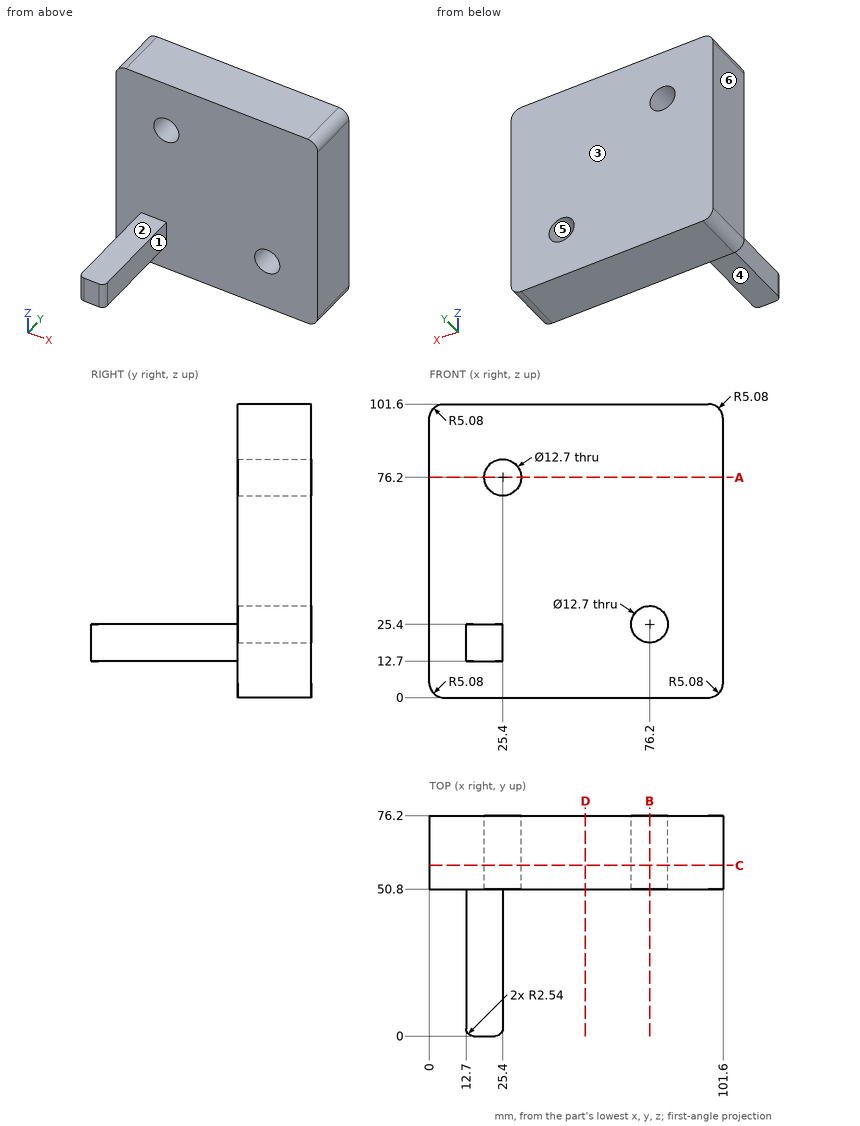
For this review, use the dimensioned drawing (mm, ordinates from the lowest corner) and the shaded views. A direction names the side the tool comes from. Round coordinates to 2 decimals unless told otherwise and drop trailing zeros. Loops run counter-clockwise (first coordinate to the right, second up) from the corner with the lowest first, then second, coordinate; pieces in that order, holes last. Notation, with made-up numbers: (-30.5, 77) -> (-7.5, 77) arc R15 ccw to (-7.5, 102) -> close; hole circle Ø3 at (-37.5, -32). An arc over 180 degrees is marked (long way). Write item = value, one per line. Start each with the question number.
Item 1: To check wall thickness, follow L1, parallel to Z at x = 76, y = 57; L2, parallel to Z at x = 25, y = 66; L3, parallel to Y at x = 79.5, z = 85. State the ranges of each line that lie inside material, in increasing order.
Item 2: For the marked faces 1, 2 and 3, list the 3-axis set-ups (+Z, -Z, +X, -X, +Y, -Y) from which the entire face can be reached by the end or side of a thin tool; tool diameter is ignored.
Item 3: Insertion check: pin 1 (12 mm diameter, centred on x = 85, z = 42, fed in from -Y); pin 2 (10 mm diameter, centred on x = 17.5, y = 24.5, fed in from +Z); pin 3 (10 mm diameter, centred on y = 33, z = 20, fed in from +X); pin 4 (10 mm diameter, centred on x = 76.2, z = 25.4, fed in from -Y). Each pin has a flat end and moves straight along its axis. Give the tip position at first contact, or say it passes through.
Item 4: Take a section at C-C on y = 59. Give the boundary of the cut face in (x, z), plus the area to 3 significant figures.
Item 5: Take a section at B-B on x = 76.2. Give the boundary of the cut face in (y, z), plus the area to 3 significant figures.
Item 6: Take a section at D-D on x = 54. Give the boundary of the cut face in (y, z).
Item 7: Take a section at A-A on z = 76.2. Give the boundary of the cut face in (x, y).
Item 8: Mouldability with a two-part tool opening along X and no side actions: class the marked faces 4, 5 and 6 as released by +X, released by -X, zero draft, split by the parting line, or undercut.
Result:
q1.L1 = 0 to 19.05, 31.75 to 101.6
q1.L2 = 0 to 69.86, 82.54 to 101.6
q1.L3 = 50.8 to 76.2
q2.face_1 = +Z, -Z, +X, -Y
q2.face_2 = +Z, +X, -X, -Y
q2.face_3 = +Z, -Z, +X, -X, +Y
q3.pin_1 = 50.8
q3.pin_2 = 25.4
q3.pin_3 = 25.4
q3.pin_4 = through
q4.outline = (0, 5.08) arc R5.08 ccw to (5.08, 0) -> (96.52, 0) arc R5.08 ccw to (101.6, 5.08) -> (101.6, 96.52) arc R5.08 ccw to (96.52, 101.6) -> (5.08, 101.6) arc R5.08 ccw to (0, 96.52) -> close; hole circle Ø12.7 at (25.4, 76.2); hole circle Ø12.7 at (76.2, 25.4)
q4.area = 10,000 mm²
q5.outline = (50.8, 0) -> (76.2, 0) -> (76.2, 19.05) -> (50.8, 19.05) -> close; (50.8, 31.75) -> (76.2, 31.75) -> (76.2, 101.6) -> (50.8, 101.6) -> close
q5.area = 2,260 mm²
q6.outline = (50.8, 0) -> (76.2, 0) -> (76.2, 101.6) -> (50.8, 101.6) -> close
q7.outline = (0, 50.8) -> (19.05, 50.8) -> (19.05, 76.2) -> (0, 76.2) -> close; (31.75, 50.8) -> (101.6, 50.8) -> (101.6, 76.2) -> (31.75, 76.2) -> close
q8.face_4 = zero draft
q8.face_5 = undercut
q8.face_6 = released by -X
